from build123d import *

# Parameters (mm, degrees)
SKETCH1_W                 = 52
SKETCH1_H                 = 66
BOSS_EXTRUDE1_DEPTH       = 6
SKETCH2_W                 = 42.5
SKETCH2_H                 = 42.5
CUT_EXTRUDE1_DEPTH        = 3
SKETCH3_R                 = 1.5
CUT_EXTRUDE2_DEPTH        = 13
SKETCH4_W                 = 10
SKETCH4_H                 = 6
BOSS_EXTRUDE2_DEPTH       = 63
SKETCH5_W                 = 4
SKETCH5_H                 = 6
BOSS_EXTRUDE3_DEPTH       = 10
SKETCH6_R                 = 0.75
CUT_EXTRUDE3_DEPTH        = 114
BOSS_EXTRUDE4_START       = -3
BOSS_EXTRUDE4_OUTLINE_W   = 78.5
BOSS_EXTRUDE4_OUTLINE_H   = 57.5
BOSS_EXTRUDE4_OUTLINE_R   = 1.5
BOSS_EXTRUDE4_DEPTH       = 3
BOSS_EXTRUDE4_START_2     = -30
BOSS_EXTRUDE4_2_OUTLINE_R = 0.75
BOSS_EXTRUDE4_2_DEPTH     = 4
BOSS_EXTRUDE4_START_3     = 55.6
BOSS_EXTRUDE4_3_OUTLINE_R = 0.75
BOSS_EXTRUDE4_3_DEPTH     = 4
SKETCH8_W                 = 52
SKETCH8_H                 = 1.5
BOSS_EXTRUDE5_DEPTH       = 6
FILLET1_R                 = 2


# Read off the part's stored shape, not the designer's step: Boss-Extrude4
with BuildPart() as part:
    # Sketch1 → Boss-Extrude1 (new body)
    with BuildSketch(Plane(origin=(0, 0, 0), x_dir=(1, 0, 0), z_dir=(0, 1, 0))):
        with Locations((-26, -33)):
            Rectangle(SKETCH1_W, SKETCH1_H)
    extrude(amount=BOSS_EXTRUDE1_DEPTH)

    # Sketch2 → Cut-Extrude1 (cut)
    with BuildSketch(Plane(origin=(0, 6, 0), x_dir=(1, 0, 0), z_dir=(0, 1, 0))):
        with Locations((-26, -33)):
            Rectangle(SKETCH2_W, SKETCH2_H)
    extrude(amount=-CUT_EXTRUDE1_DEPTH, mode=Mode.SUBTRACT)

    # Sketch3 → Cut-Extrude2 (cut)
    with BuildSketch(Plane(origin=(0, 6, 0), x_dir=(1, 0, 0), z_dir=(0, 1, 0))):
        with Locations(Location((-42.25, -3.75, 0), (0, 0, 270))):
            Circle(SKETCH3_R)
        with Locations(Location((-9.75, -3.75, 0), (0, 0, 90))):
            Circle(SKETCH3_R)
        with Locations(Location((-9.75, -62.25, 0), (0, 0, 270))):
            Circle(SKETCH3_R)
        with Locations(Location((-42.25, -62.25, 0), (0, 0, 90))):
            Circle(SKETCH3_R)
    extrude(amount=-CUT_EXTRUDE2_DEPTH, mode=Mode.SUBTRACT)

    # Sketch4 → Boss-Extrude2 (add)
    with BuildSketch(Plane(origin=(0, 0, 0), x_dir=(0, 0, -1), z_dir=(1, 0, 0))):
        with Locations((-5, 3)):
            Rectangle(SKETCH4_W, SKETCH4_H)
    extrude(amount=BOSS_EXTRUDE2_DEPTH)

    # Sketch5 → Boss-Extrude3 (add)
    with BuildSketch(Plane(origin=(0, 0, 0), x_dir=(-1, 0, 0), z_dir=(0, 0, -1))):
        with Locations((28, 3)):
            Rectangle(SKETCH5_W, SKETCH5_H)
        with Locations((-57.6, 3)):
            Rectangle(SKETCH5_W, SKETCH5_H)
    extrude(amount=BOSS_EXTRUDE3_DEPTH)

    # Sketch6 → Cut-Extrude3 (cut)
    with BuildSketch(Plane(origin=(59.6, 0, 0), x_dir=(0, 0, -1), z_dir=(1, 0, 0))):
        with Locations((4, 1.5)):
            Circle(SKETCH6_R)
    extrude(amount=-CUT_EXTRUDE3_DEPTH, mode=Mode.SUBTRACT)

    # Boss-Extrude4 outline → Boss-Extrude4 (add)
    with BuildSketch(Plane(origin=(0, 0, 0), x_dir=(-1, 0, 0), z_dir=(0, -1, 0)).offset(BOSS_EXTRUDE4_START)):
        with Locations((-39.25, -38.75)):
            Rectangle(BOSS_EXTRUDE4_OUTLINE_W, BOSS_EXTRUDE4_OUTLINE_H)
        with Locations((-74.5, -63.5)):
            Circle(BOSS_EXTRUDE4_OUTLINE_R, mode=Mode.SUBTRACT)
        with Locations((-74.5, -14)):
            Circle(BOSS_EXTRUDE4_OUTLINE_R, mode=Mode.SUBTRACT)
    extrude(amount=BOSS_EXTRUDE4_DEPTH)

    # Boss-Extrude4 2 outline → Boss-Extrude4 2 (add)
    with BuildSketch(Plane.YZ.offset(BOSS_EXTRUDE4_START_2)):
        with Locations((1.5, -4)):
            Circle(BOSS_EXTRUDE4_2_OUTLINE_R)
    extrude(amount=BOSS_EXTRUDE4_2_DEPTH)

    # Boss-Extrude4 3 outline → Boss-Extrude4 3 (add)
    with BuildSketch(Plane.YZ.offset(BOSS_EXTRUDE4_START_3)):
        with Locations((1.5, -4)):
            Circle(BOSS_EXTRUDE4_3_OUTLINE_R)
    extrude(amount=BOSS_EXTRUDE4_3_DEPTH)

    # Sketch8 → Boss-Extrude5 (add)
    with BuildSketch(Plane(origin=(0, 0, 0), x_dir=(-1, 0, 0), z_dir=(0, -1, 0))):
        with Locations((26, -66.75)):
            Rectangle(SKETCH8_W, SKETCH8_H)
    extrude(amount=-BOSS_EXTRUDE5_DEPTH)

    # Fillet1
    fillet1_edges = [part.edges().sort_by_distance(p)[0] for p in [
        (-52, 6, 33.75),
        (-26, 6, 67.5),
        (0, 6, 38.75),
        (31.5, 6, 10),
        (63, 6, 5),
        (-41, 6, 0),
        (14.8, 6, 0),
    ]]
    fillet(fillet1_edges, radius=FILLET1_R)


solid = part.part
Here's how the part is built. I have some questions about the finished solid (model axes, mm). A direction names the side the tool comes from. Round coordinates to 2 decimals unless told otherwise and drop trailing zeros. Loops run counter-clockwise (first coordinate to the right, second up) from the corner with the lowest first, then second, coordinate; pieces in that order, holes last.
1. If we section it at B-B on x = 74.5: Write out the boundary of the cut face in (y, z).
Answer list:
outline: (0, 10) - (3, 10) - (3, 12.5) - (0, 12.5) - close; (0, 15.5) - (3, 15.5) - (3, 62) - (0, 62) - close; (0, 65) - (3, 65) - (3, 67.5) - (0, 67.5) - close
2. If we section it at A-A on y = 2.1: Write out the boundary of the cut face in (x, z).
Answer list:
outline: (-52, 0) - (-30, 0) - (-30, -10) - (-26, -10) - (-26, 0) - (55.6, 0) - (55.6, -10) - (59.6, -10) - (59.6, 0) - (63, 0) - (63, 10) - (78.5, 10) - (78.5, 67.5) - (-52, 67.5) - close; hole circle Ø3 at (-42.25, 3.75); hole circle Ø3 at (-42.25, 62.25); hole circle Ø3 at (-9.75, 3.75); hole circle Ø3 at (-9.75, 62.25); hole circle Ø3 at (74.5, 14); hole circle Ø3 at (74.5, 63.5)
3. If I drill on line 1 along Z through (x, y) = (74.5, 2.2); line 2 along X through (y, z) = (3.25, 62.25); line 3 along X through (y, z) = (2, 3.75), over which ranges is the centre line in solid material (lowest first)?
Answer list:
line 1: z = 10 to 12.5, 15.5 to 62, 65 to 67.5
line 2: x = -52 to -43.75, -40.75 to -11.25, -8.25 to 0
line 3: x = -52 to -43.75, -40.75 to -11.25, -8.25 to 63
4. If we section it at D-D on z = 3.75: Write out the boundary of the cut face in (x, y).
Answer list:
outline: (-52, 0) - (-43.75, 0) - (-43.75, 6) - (-50, 6) arc R2 ccw to (-52, 4) - close; (-40.75, 0) - (-11.25, 0) - (-11.25, 6) - (-40.75, 6) - close; (-8.25, 0) - (63, 0) - (63, 4) arc R2 ccw to (61, 6) - (-8.25, 6) - close
5. If we section it at C-C on z = 36: Write out the boundary of the cut face in (x, y), plus the area to 3 significant figures.
Answer list:
outline: (-52, 0) - (78.5, 0) - (78.5, 3) - (0, 3) - (0, 4) arc R2 ccw to (-2, 6) - (-4.75, 6) - (-4.75, 3) - (-47.25, 3) - (-47.25, 6) - (-50, 6) arc R2 ccw to (-52, 4) - close
area: 418 mm2
6. For P1, Ø2.5, axis at x = 71.5, y = 1.5, coming from the -Z side; P2, Ø2, axis at x = 54, z = 36, coming from the +Y side; P3, Ø3, axis at x = -39.5, y = 3, coming from the -Z side, each with a flat end and sliding along its axis, tell me the tip position at first contact or that it passes through.
Answer list:
P1: stops at z = 10
P2: stops at y = 3
P3: stops at z = 0
7. We'd pull the mould along Z, two halves only. Please class faces 4 (the face through (14, 2, 67.5)), 5 (the face through (59.6, 3, -5)), 6 (the face through (14, 2, 0)), 7 (the face through (-10.325, 3.042, 63.636)): +Z half, -Z half, draft (parallel to the pull), parting line (faces both ways), or undercut.
Answer list:
face 4: +Z half
face 5: draft
face 6: -Z half
face 7: undercut
8. Which directions (+Z, -Z, +X, -X, +Y, -Y) give clear straight access to the entire face, cutting with the end or side of a thin tool? Please do faces 1 (the face through (-26, 3, 33)), 2 (the face through (71, 2, 10)), 3 (the face through (40, 3, 38)).
Answer list:
face 1: +Y
face 2: -Z, +X, +Y, -Y
face 3: +Z, +X, +Y
